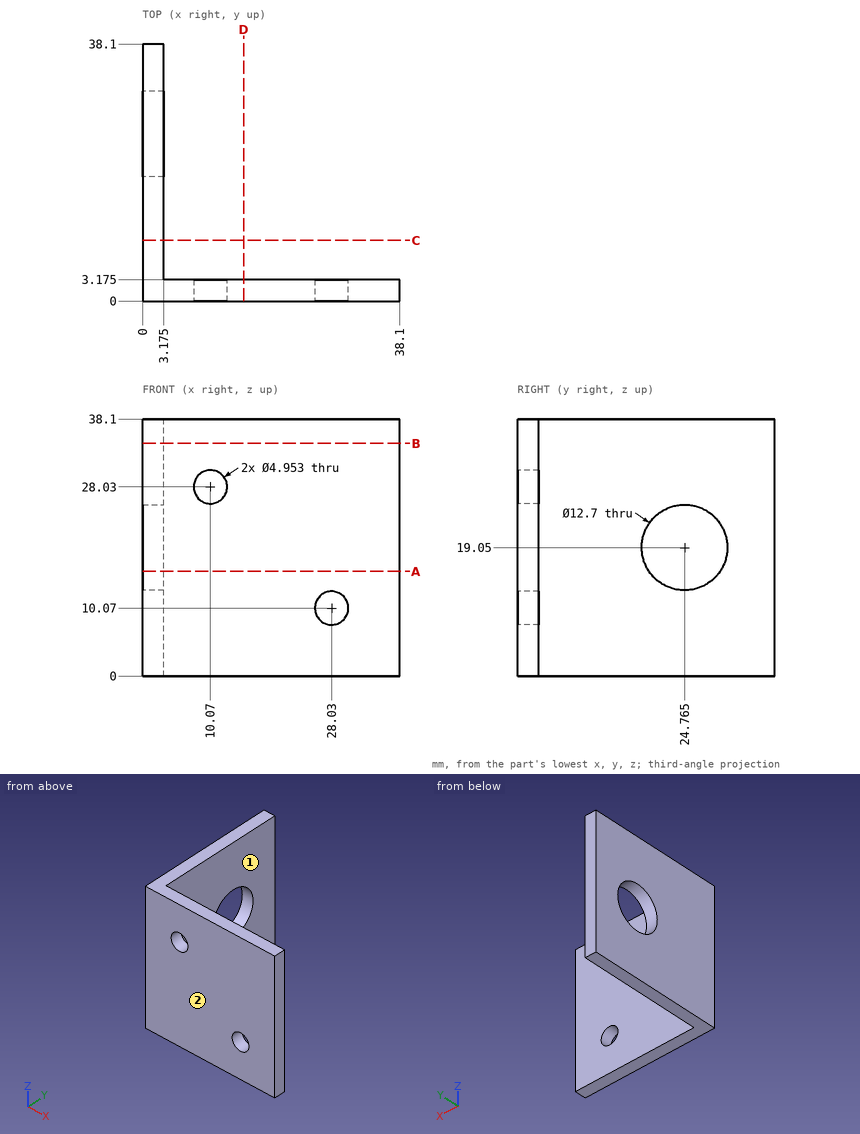
Geometry: see drawing. Coordinates: mm, zero at the bounding-box minimum. A direction names the side the tool comes from. Give positions to 0.01 mm unless a question says otherwise; leave off trailing zeros. Order: outer loops, then holes, each group sorted by start corner. A loop starts at its lowest first (then second) coordinate and runs counter-clockwise, first axis right, second up. Notation, with made-up numbers: (37, -13.75) - (83, -13.75) arc R33 cw to (83, 16.25) - close; hole circle Ø11 at (-22, 15.25). An arc over 180 degrees is marked (long way). One line per item, written item: value.
1. Pin query (flat end, axial travel): pin 1 Ø10.5 at (y, z) = (28, 17.5) entering from +X (3 decimals); pin 2 Ø10 at (y, z) = (24.765, 19.05) entering from -X; pin 3 Ø10.5 at (x, z) = (14, 11.5) entering from +Y (3 decimals). Return the tip coordinate at first contact, or that it passes through.
Determined:
pin 1: x = 3.175
pin 2: through
pin 3: y = 3.175
2. Cut plane B-B, the plane z = 34.5. Output: boundary loops of the cut face in (x, y) (1 decimal), and give its area (3 significant figures).
Determined:
outline: (0, 0) - (38.1, 0) - (38.1, 3.2) - (3.2, 3.2) - (3.2, 38.1) - (0, 38.1) - close
area: 232 mm2
3. Reachability of the marked faces 1 and 2 from +Z, -Z, +X, -X, +Y, -Y: full face, straight path, thin tool, end or side. Return the list, or none.
Determined:
face 1: +Z, -Z, +X, +Y
face 2: +Z, -Z, +X, -X, -Y
4. Cut plane A-A, the plane z = 15.5. Output: boundary loops of the cut face in (x, y) (1 decimal).
Determined:
outline: (0, 0) - (38.1, 0) - (38.1, 3.2) - (3.2, 3.2) - (3.2, 19.5) - (0, 19.5) - close; (0, 30) - (3.2, 30) - (3.2, 38.1) - (0, 38.1) - close
5. Cut plane C-C, the plane y = 9. Output: boundary loops of the cut face in (x, z) (1 decimal).
Determined:
outline: (0, 0) - (3.2, 0) - (3.2, 38.1) - (0, 38.1) - close
6. Line query: probe 1 along Y at (x, z) = (1.05, 19.05) (1 decimal); probe 2 along Y at (x, z) = (32.5, 31.5) (1 decimal). Output: solid intervals per line, ascending.
Determined:
probe 1: 0 to 18.4, 31.1 to 38.1
probe 2: 0 to 3.2
